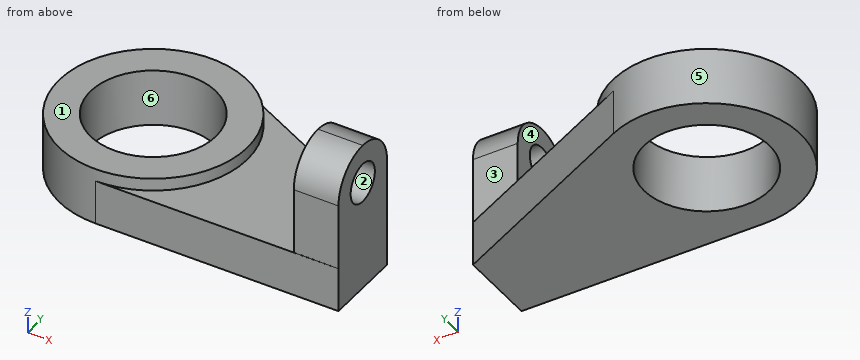
```python
from build123d import *

# Parameters (mm, degrees)
SKETCH_1_R          = 52.5
SKETCH_1_R_2        = 35
EXTRUDE_1_DEPTH     = 32
EXTRUDE_3_DEPTH     = 25
SKETCH_3_W          = 25
SKETCH_3_H          = 44
EXTRUDE_4_DEPTH     = 59
FILLET_1_R          = 22
SKETCH_4_R          = 11
CUT_EXTRUDE_1_DEPTH = 59


with BuildPart() as part:
    # 스케치1 → 보스-돌출1 (new body)
    with BuildSketch(Plane.XY):
        Circle(SKETCH_1_R)
        Circle(SKETCH_1_R_2, mode=Mode.SUBTRACT)
    extrude(amount=EXTRUDE_1_DEPTH)

    # 스케치2 → 보스-돌출3 (add)
    with BuildSketch(Plane(origin=(0, 0, 0), x_dir=(-1, 0, 0), z_dir=(0, 0, -1))):
        with BuildLine():
            Line((-23.122008196, 47.134093149), (-135.758979711, -8.120878455))
            Line((-135.758979711, -8.120878455), (-135.758979711, -52.120878455))
            Line((-135.758979711, -52.120878455), (-0.146690573, -52.499795065))
            ThreePointArc((-0.146690573, -52.499795065), (-51.157462855, -11.796778977), (-23.122008196, 47.134093149))
        make_face()
    extrude(amount=-EXTRUDE_3_DEPTH)

    # 스케치3 → 보스-돌출4 (add)
    with BuildSketch(Plane.XY.offset(25)):
        with Locations((123.258979711, -30.120878455)):
            Rectangle(SKETCH_3_W, SKETCH_3_H)
    extrude(amount=EXTRUDE_4_DEPTH)

    # 필렛1
    fillet_1_edges = [part.edges().sort_by_distance(p)[0] for p in [
        (123.258979711, -8.120878455, 84),
        (123.258979711, -52.120878455, 84),
    ]]
    fillet(fillet_1_edges, radius=FILLET_1_R - 0.0001)  # a hair under: the kernel refuses the full size

    # 스케치4 → 컷-돌출1 (cut)
    with BuildSketch(Plane.ZY.offset(-110.758979711)):
        with Locations((62, -30.120878455)):
            Circle(SKETCH_4_R)
    extrude(amount=-CUT_EXTRUDE_1_DEPTH, mode=Mode.SUBTRACT)


solid = part.part
```
Work out the finished part from the listing and answer in its coordinate system (mm). Face numbers are marked on the shaded views. A direction names the side the tool comes from. Coordinates: 2 decimals unless noted, no trailing zeros. Loops run counter-clockwise (first coordinate to the right, second up) from the corner with the lowest first, then second, coordinate; pieces in that order, holes last.
1) Section C-C (z = 12) is taken. Give the vertices of the cut face in (x, y).
Results:
outline: (0.15, -52.5) - (135.76, -52.12) - (135.76, -8.12) - (23.12, 47.13) arc R52.5 ccw (long way) to start; hole circle Ø70 at (0, 0)
2) For the marked faces 1, 2 and 3, determine the directions among +Z, -Z, +X, -X, +Y, -Y from which every point of the face is accessible in a straight line to the end or side of a thin tool.
Results:
face 1: +Z, -X, +Y, -Y
face 2: +X, -X
face 3: +Z, +X, +Y
3) Section B-B (y = -33) is taken. Give the vertices of the cut face in (x, z).
Results:
outline: (-40.83, 0) - (-11.66, 0) - (-11.66, 32) - (-40.83, 32) - close; (11.66, 0) - (135.76, 0) - (135.76, 51.38) - (110.76, 51.38) - (110.76, 25) - (40.83, 25) - (40.83, 32) - (11.66, 32) - close; (110.76, 72.62) - (135.76, 72.62) - (135.76, 83.81) - (110.76, 83.81) - close
4) Section A-A (z = 29.5) is taken. Give the vertices of the cut face in (x, y), plus the area to 3 significant figures.
Results:
outline: circle Ø105 at (0, 0); (110.76, -52.12) - (135.76, -52.12) - (135.76, -8.12) - (110.76, -8.12) - close; hole circle Ø70 at (0, 0)
area: 5,910 mm2
5) Consider probe 1 along Y at (x, z) = (118.75, 62); probe 2 along Y at (x, z) = (0, 17); probe 3 along Z at (x, y) = (27, -29.5). Determine where each line is inside the solid, lowest interval first.
Results:
probe 1: y = -52.12 to -41.12, -19.12 to -8.12
probe 2: y = -52.5 to -35, 35 to 52.5
probe 3: z = 0 to 32
6) Flat-ended cylindrical pins translate along their axes: pin 1 (12.5 mm diameter, centred on x = 126.5, z = 36.5, fed in from +Y); pin 2 (1.5 mm diameter, centred on y = 30.5, z = 22, fed in from -X); pin 3 (10 mm diameter, centred on x = 51, y = -35, fed in from +Z). Find the tip coordinate at first contact, or state that the pin passes through.
Results:
pin 1: stops at y = -8.12
pin 2: stops at x = -43.26
pin 3: stops at z = 25
7) Section D-D (x = -18) is taken. Give the vertices of the cut face in (y, z).
Results:
outline: (-49.32, 0) - (-30.02, 0) - (-30.02, 32) - (-49.32, 32) - close; (30.02, 0) - (49.32, 0) - (49.32, 32) - (30.02, 32) - close
8) For a pull along Y with two mould halves and no side action, classify the marked faces 4, 5 and 6 as +Y half, -Y half, draft (parallel to the pull), parting line (faces both ways), or undercut.
Results:
face 4: draft
face 5: parting line
face 6: undercut
